For this review, take the finished solid that the model builds, in its own axes (mm). A direction names the side the tool comes from. Coordinates: 2 decimals unless noted, no trailing zeros. Write each loop counter-clockwise with the first axis right and the second up, starting at its lowest first coordinate (ties: lowest second). Pieces come first, ordered by that corner, then holes.
```python
from build123d import *

# Parameters (mm, degrees)
F1_DEPTH = 19.05
F2_DEPTH = 12.7
F3_DEPTH = 19.05


with BuildPart() as f1:
    # F0 (on Top) → F1 (new body)
    with BuildSketch(Plane.XY):
        Polygon((-170.413183, 61.813528), (-178.363383, 53.863328), (-178.363383, -68.348772), (-170.413183, -76.298972), (142.298917, -76.298972), (150.249117, -68.348772), (150.249117, 53.876028), (142.311617, 61.813528), align=None)
    extrude(amount=F1_DEPTH)

    # F0 (on Top) → F2 (join)
    with BuildSketch(Plane.XY):
        Polygon((153.424117, 53.876028), (142.311617, 64.988528), (-170.413183, 64.988528), (-181.538383, 53.863328), (-181.538383, -68.348772), (-170.413183, -79.473972), (142.298917, -79.473972), (153.424117, -68.348772), align=None)
        Polygon((-178.363383, -68.348772), (-178.363383, 53.863328), (-170.413183, 61.813528), (142.311617, 61.813528), (150.249117, 53.876028), (150.249117, -68.348772), (142.298917, -76.298972), (-170.413183, -76.298972), align=None, mode=Mode.SUBTRACT)
    extrude(amount=F2_DEPTH)

    # F0 (on Top) → F3 (join)
    with BuildSketch(Plane.XY):
        with BuildLine():
            Line((178.824117, 53.876028), (142.311617, 90.388528))
            Line((142.311617, 90.388528), (-170.413183, 90.388528))
            Line((-170.413183, 90.388528), (-206.938383, 53.863328))
            Line((-206.938383, 53.863328), (-206.938383, -68.348772))
            Line((-206.938383, -68.348772), (-170.413183, -104.873972))
            Line((-170.413183, -104.873972), (-90.257133, -104.873972))
            ThreePointArc((-90.257133, -104.873972), (-14.057133, -140.022369), (62.142867, -104.873972))
            Line((62.142867, -104.873972), (142.298917, -104.873972))
            Line((142.298917, -104.873972), (178.824117, -68.348772))
            Line((178.824117, -68.348772), (178.824117, 53.876028))
        make_face()
        Polygon((-170.413183, 64.988528), (142.311617, 64.988528), (153.424117, 53.876028), (153.424117, -68.348772), (142.298917, -79.473972), (-170.413183, -79.473972), (-181.538383, -68.348772), (-181.538383, 53.863328), align=None, mode=Mode.SUBTRACT)
    extrude(amount=F3_DEPTH)


solid = f1.part
```
Q1. Add section C-C (y = -93.5). State the section outline as (x, z) points, then the cut area to 3 significant figures.
Ans:
outline: (-181.79, 0) - (153.67, 0) - (153.67, 19.05) - (-181.79, 19.05) - close
area: 6,390 mm2
Q2. Clearance check with flat-ended pins moving along their axes: pin 1 Ø5.5 at (x, z) = (118, 12.5) entering from -Y; pin 2 Ø3 at (x, y) = (104, -35.5) entering from -Z; pin 3 Ø5 at (y, z) = (56.5, 15.5) entering from -X; pin 4 Ø7 at (x, z) = (0, 14.5) entering from -Y. State where each tip first meets the part, or that it passes through.
Ans:
pin 1: stops at y = -104.87
pin 2: stops at z = 0
pin 3: stops at x = -206.8
pin 4: stops at y = -139.46
Q3. Draft analysis for pull direction Y (two halves, no side actions). For faces 1 (the flat face through (160.306, -86.867, 9.392)), 2 (the flat face through (-27.2, -76.5, 12.7)), 3 (the flat face through (-188.4, 72.4, 9.4)), state which applies: +Y half, -Y half, draft (parallel to the pull), parting line (faces both ways), or undercut.
Ans:
face 1: -Y half
face 2: undercut
face 3: +Y half
Q4. Add section A-A (x = 127). State the section outline as (y, z) points, then the cut area to 3 significant figures.
Ans:
outline: (-104.87, 0) - (90.39, 0) - (90.39, 19.05) - (64.99, 19.05) - (64.99, 12.7) - (61.81, 12.7) - (61.81, 19.05) - (-76.3, 19.05) - (-76.3, 12.7) - (-79.47, 12.7) - (-79.47, 19.05) - (-104.87, 19.05) - close
area: 3,680 mm2
Q5. Add section D-D (x = -70). State the section outline as (y, z) points.
Ans:
outline: (-122.95, 0) - (90.39, 0) - (90.39, 19.05) - (64.99, 19.05) - (64.99, 12.7) - (61.81, 12.7) - (61.81, 19.05) - (-76.3, 19.05) - (-76.3, 12.7) - (-79.47, 12.7) - (-79.47, 19.05) - (-122.95, 19.05) - close
Q6. Tool access review of faces 4 (the flat face through (146.2, -72.4, 15.8)), 5 (the flat face through (178.824, -8, 9)), 6 (the flat face through (102, -104.874, 9)): name each direction out of +Z, -Z, +X, -X, +Y, -Y from which nothing blocks a thin tool from reaching the whole face with its end or side.
Ans:
face 4: +Z
face 5: +Z, -Z, +X, +Y, -Y
face 6: +Z, -Z, +X, -Y
Q7. For probe 1 along Y at (x, z) = (-120, 4.75); probe 2 along Z at (x, y) = (-17, -77); probe 3 along Y at (x, z) = (158, 8.25), list the stretches that pass through material, from the lowest coordinate up.
Ans:
probe 1: y = -104.87 to 90.39
probe 2: z = 0 to 12.7
probe 3: y = -89.17 to 74.7
Q8. Add section B-B (z = 6.75). State the section outline as (x, y) points.
Ans:
outline: (-206.94, -68.35) - (-170.41, -104.87) - (-90.26, -104.87) arc R100.17 ccw to (62.14, -104.87) - (142.3, -104.87) - (178.82, -68.35) - (178.82, 53.88) - (142.31, 90.39) - (-170.41, 90.39) - (-206.94, 53.86) - close
